Verification items for the finished model (mm, model axes). Face numbers are marked on the shaded views. A direction names the side the tool comes from. Round coordinates to 2 decimals unless told otherwise and drop trailing zeros. Order: outer loops, then holes, each group sorted by start corner. A loop starts at its lowest first (then second) coordinate and runs counter-clockwise, first axis right, second up. Notation, with made-up numbers: (88, -22) -> (130, -22) arc R8 ccw to (130, -8) -> close; hole circle Ø9 at (81, 20). An arc over 180 degrees is marked (long way). Return JSON: item names as keys, results as strings. Group by question number.
1) Tool access check on the marked faces 1 and 2. Record the directions out of +Z, -Z, +X, -X, +Y, -Y that give a thin tool (end or side, any length) a straight path to the whole face; none if there is none.
2) Scan lines: L1, parallel to X at y = -8, z = 85.5; L2, parallel to Y at x = 46.5, z = 56; L3, parallel to X at y = 4.75, z = 279.4. Record each from-to range of solid material in increasing order.
3) Section check B-B on x = 17. Enter the section's corners in (y, z).
4) Depth check by flat-ended pin: pin 1 (4 mm diameter, centred on x = 8.58, z = 279.4, fed in from -Y); pin 2 (2.5 mm diameter, centred on x = 99.38, z = 6.35, fed in from +Y); pin 3 (3.5 mm diameter, centred on x = -76, z = 267.5, fed in from +Y); pin 4 (1 mm diameter, centred on x = 61, y = -1, fed in from -Z). Enter the tip coordinate at first touch or a pass-through.
5) Section check A-A on z = 156. Enter the section's corners in (x, y), plus the area to 3 significant figures.
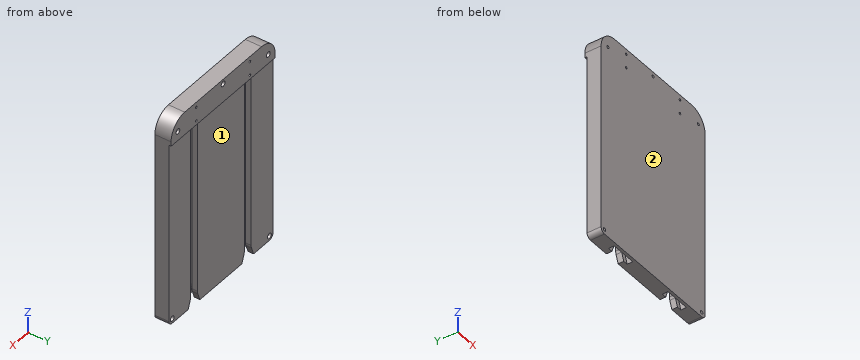
```python
from build123d import *
from OCP.BRepFilletAPI import BRepFilletAPI_MakeChamfer

# Parameters (mm, degrees)
BOSS_EXTRUDE1_DEPTH                            = 254
SKETCH2_W                                      = 194.31
SKETCH2_H                                      = 44.45
SKETCH2_W_2                                    = 35.56
SKETCH2_H_2                                    = 17.018
BOSS_EXTRUDE2_DEPTH                            = 6.35
BOSS_EXTRUDE3_DEPTH                            = 44.45
CUT_EXTRUDE1_DEPTH                             = 324.390875065
CUT_EXTRUDE1_DEPTH_BACK                        = 324.390875065
SKETCH5_R                                      = 1.524
FILLET1_R                                      = 3.175
FILLET2_R                                      = 3.175
CBORE_FOR_6_SOCKET_HEAD_CAP_SCREW1_D           = 4.3053
CBORE_FOR_6_SOCKET_HEAD_CAP_SCREW1_CBORE_D     = 7.14502
CBORE_FOR_6_SOCKET_HEAD_CAP_SCREW1_CBORE_DEPTH = 3.5052
CHAMFER1_SIZE                                  = 12.7
CHAMFER1_SIZE2                                 = 4.622421975
FILLET4_R                                      = 12.7
FILLET6_R                                      = 6.35
FILLET7_R                                      = 2.54
CUT_EXTRUDE2_DEPTH                             = 363.564005121
SKETCH13_W                                     = 19.143193239
SKETCH13_H                                     = 43.092698141
CUT_EXTRUDE3_DEPTH                             = 362.835089653
FILLET8_R                                      = 25.4
CBORE_FOR_6_SOCKET_HEAD_CAP_SCREW3_D           = 3.6576
CBORE_FOR_6_SOCKET_HEAD_CAP_SCREW3_CBORE_D     = 7.14502
CBORE_FOR_6_SOCKET_HEAD_CAP_SCREW3_CBORE_DEPTH = 3.5052
CBORE_FOR_6_SOCKET_HEAD_CAP_SCREW4_D           = 3.6576
CBORE_FOR_6_SOCKET_HEAD_CAP_SCREW4_CBORE_D     = 7.14502
CBORE_FOR_6_SOCKET_HEAD_CAP_SCREW4_CBORE_DEPTH = 3.5052


with BuildPart() as part:
    # Sketch1 → Boss-Extrude1 (new body)
    with BuildSketch(Plane.XY):
        Polygon((-88.579180599, 2.764546242), (-47.939180599, 2.764546242), (-47.939180599, -4.855453758), (-54.289180599, -4.855453758), (-54.289180599, -12.475453758), (-28.889180599, -12.475453758), (-28.889180599, -4.855453758), (-35.239180599, -4.855453758), (-35.239180599, 2.764546242), (5.400819401, 2.764546242), (5.400819401, 28.164546242), (11.750819401, 28.164546242), (11.750819401, 2.764546242), (52.390819401, 2.764546242), (52.390819401, -4.855453758), (46.040819401, -4.855453758), (46.040819401, -12.475453758), (71.440819401, -12.475453758), (71.440819401, -4.855453758), (65.090819401, -4.855453758), (65.090819401, 2.764546242), (105.730819401, 2.764546242), (105.730819401, -16.285453758), (-88.579180599, -16.285453758), align=None)
    extrude(amount=BOSS_EXTRUDE1_DEPTH)

    # Sketch2 → Boss-Extrude2 (add)
    with BuildSketch(Plane.XY.offset(254)):
        with Locations((8.575819401, 5.939546242)):
            Rectangle(SKETCH2_W, SKETCH2_H)
        with Locations((-41.589180599, 14.321546242)):
            Rectangle(SKETCH2_W_2, SKETCH2_H_2, mode=Mode.SUBTRACT)
        with Locations((58.740819401, 14.321546242)):
            Rectangle(SKETCH2_W_2, SKETCH2_H_2, mode=Mode.SUBTRACT)
    extrude(amount=BOSS_EXTRUDE2_DEPTH)

    # Sketch3 → Boss-Extrude3 (add)
    with BuildSketch(Plane.XY.offset(260.35)):
        Polygon((-88.579180599, 5.812546242), (-88.579180599, -16.285453758), (105.730819401, -16.285453758), (105.730819401, 5.812546242), (76.520819401, 5.812546242), (40.960819401, 5.812546242), (-23.809180599, 5.812546242), (-59.369180599, 5.812546242), align=None)
    extrude(amount=BOSS_EXTRUDE3_DEPTH)

    # Sketch5 → Cut-Extrude1 (cut, two sides: drawn at the far end of the back side and taken through both)
    with BuildSketch(Plane(origin=(0, 5.812546242, 0), x_dir=(1, 0, 0), z_dir=(0, 1, 0)).offset(-CUT_EXTRUDE1_DEPTH_BACK)):
        with Locations(Location((-41.589180599, -259.614, 0), (0, 0, 180))):
            Circle(SKETCH5_R)
        with Locations(Location((-41.589180599, -278.664, 0), (0, 0, 180))):
            Circle(SKETCH5_R)
        with Locations(Location((58.740819401, -259.614, 0), (0, 0, 180))):
            Circle(SKETCH5_R)
        with Locations(Location((58.740819401, -278.664, 0), (0, 0, 180))):
            Circle(SKETCH5_R)
    extrude(amount=CUT_EXTRUDE1_DEPTH + CUT_EXTRUDE1_DEPTH_BACK, mode=Mode.SUBTRACT)

    # Fillet1
    # the kernel refuses this fillet: 3.175 mm, written as the material it takes off along each edge
    with BuildSketch(Plane(origin=(5.400819401, 28.164546242, -7.9375), x_dir=(0, -1, 0), z_dir=(0, 0, 1))) as fillet1_piece_1:
        with BuildLine():
            CenterArc((FILLET1_R, FILLET1_R), FILLET1_R, 180, 90)
            Line((0, FILLET1_R), (0, 0))
            Line((0, 0), (FILLET1_R, 0))
        make_face()
    extrude(amount=261.9375, mode=Mode.SUBTRACT)
    with BuildSketch(Plane(origin=(11.750819401, 28.164546242, -7.9375), x_dir=(0, -1, 0), z_dir=(0, 0, 1))) as fillet1_piece_2:
        with BuildLine():
            CenterArc((FILLET1_R, -FILLET1_R), FILLET1_R, 90, 90)
            Line((0, -FILLET1_R), (0, 0))
            Line((0, 0), (FILLET1_R, 0))
        make_face()
    extrude(amount=261.9375, mode=Mode.SUBTRACT)

    # Fillet2
    # the kernel refuses this fillet: 3.175 mm, written as the material it adds along each edge
    # the kernel refuses this fillet: 3.175 mm, written as the material it takes off along each edge
    with BuildSketch(Plane(origin=(65.343823241, 28.164546242, 260.35), x_dir=(0, -1, 0), z_dir=(-1, 0, 0))) as fillet2_2_piece_1:
        with BuildLine():
            CenterArc((FILLET2_R, -FILLET2_R), FILLET2_R, 90, 90)
            Line((0, -FILLET2_R), (0, 0))
            Line((0, 0), (FILLET2_R, 0))
        make_face()
    extrude(amount=113.536007681, mode=Mode.SUBTRACT)
    with BuildSketch(Plane(origin=(113.668319401, 28.164546242, 260.35), x_dir=(0, -1, 0), z_dir=(-1, 0, 0)), Plane(origin=(-34.986176759, 28.164546242, 260.35), x_dir=(0, -1, 0), z_dir=(-1, 0, 0))) as fillet2_2_piece_2:
        with BuildLine():
            CenterArc((FILLET2_R, -FILLET2_R), FILLET2_R, 90, 90)
            Line((0, -FILLET2_R), (0, 0))
            Line((0, 0), (FILLET2_R, 0))
        make_face()
    extrude(amount=61.53050384, mode=Mode.SUBTRACT)
    with BuildSketch(Plane(origin=(-96.516680599, 28.164546242, 254), x_dir=(0, -1, 0), z_dir=(1, 0, 0))) as fillet2_2_piece_3_section:
        with BuildLine():
            CenterArc((FILLET2_R, -FILLET2_R), FILLET2_R, 90, 90)
            Line((0, -FILLET2_R), (0, 0))
            Line((0, 0), (FILLET2_R, 0))
        make_face()
    fillet2_2_piece_3 = extrude(amount=105.0925, mode=Mode.PRIVATE)
    fillet2_2_piece_3 = fillet2_2_piece_3 - Plane(origin=(8.575819401, 24.989546242, 254.709193206), x_dir=(0, -1, 0), z_dir=(0, 0, -1)) * Cylinder(3.175, 223, mode=Mode.PRIVATE)
    add(fillet2_2_piece_3, mode=Mode.SUBTRACT)

    # CBORE for #6 Socket Head Cap Screw1 (through all)
    with Locations(Plane(origin=(0, 2.764546242, 0), x_dir=(1, 0, 0), z_dir=(0, 1, 0))):
        with Locations((99.380819401, -6.35), (-82.229180599, -6.35)):
            CounterBoreHole(CBORE_FOR_6_SOCKET_HEAD_CAP_SCREW1_D / 2, CBORE_FOR_6_SOCKET_HEAD_CAP_SCREW1_CBORE_D / 2, CBORE_FOR_6_SOCKET_HEAD_CAP_SCREW1_CBORE_DEPTH)

    # Chamfer1: one chamfer whose edges measure the first distance from different faces: ONE call of the kernel's chamfer builder (chamfer() names one face for all edges)
    chamfer1_edges_1 = [part.edges().sort_by_distance(p)[0] for p in [
        (-47.939180599, -1.045453758, 0),
    ]]
    chamfer1_side_1 = [part.faces().sort_by_distance(p)[0] for p in [
        (-47.939180599, -1.045453758, 127),
    ]]
    chamfer1_edges_2 = [part.edges().sort_by_distance(p)[0] for p in [
        (-54.289180599, -8.665453758, 0),
    ]]
    chamfer1_side_2 = [part.faces().sort_by_distance(p)[0] for p in [
        (-54.289180599, -8.665453758, 127),
    ]]
    chamfer1_edges_3 = [part.edges().sort_by_distance(p)[0] for p in [
        (-28.889180599, -8.665453758, 0),
    ]]
    chamfer1_side_3 = [part.faces().sort_by_distance(p)[0] for p in [
        (-28.889180599, -8.665453758, 127),
    ]]
    chamfer1_edges_4 = [part.edges().sort_by_distance(p)[0] for p in [
        (-35.239180599, -1.045453758, 0),
    ]]
    chamfer1_side_4 = [part.faces().sort_by_distance(p)[0] for p in [
        (-35.239180599, -1.045453758, 127),
    ]]
    chamfer1_edges_5 = [part.edges().sort_by_distance(p)[0] for p in [
        (52.390819401, -1.045453758, 0),
    ]]
    chamfer1_side_5 = [part.faces().sort_by_distance(p)[0] for p in [
        (52.390819401, -1.045453758, 127),
    ]]
    chamfer1_edges_6 = [part.edges().sort_by_distance(p)[0] for p in [
        (46.040819401, -8.665453758, 0),
    ]]
    chamfer1_side_6 = [part.faces().sort_by_distance(p)[0] for p in [
        (46.040819401, -8.665453758, 127),
    ]]
    chamfer1_edges_7 = [part.edges().sort_by_distance(p)[0] for p in [
        (71.440819401, -8.665453758, 0),
    ]]
    chamfer1_side_7 = [part.faces().sort_by_distance(p)[0] for p in [
        (71.440819401, -8.665453758, 127),
    ]]
    chamfer1_edges_8 = [part.edges().sort_by_distance(p)[0] for p in [
        (65.090819401, -1.045453758, 0),
    ]]
    chamfer1_side_8 = [part.faces().sort_by_distance(p)[0] for p in [
        (65.090819401, -1.045453758, 127),
    ]]
    chamfer1 = BRepFilletAPI_MakeChamfer(part.part.solid().wrapped)
    for e in chamfer1_edges_1:
        chamfer1.Add(CHAMFER1_SIZE, CHAMFER1_SIZE2, e.wrapped, chamfer1_side_1[0].wrapped)  # the first distance lies on this face
    for e in chamfer1_edges_2:
        chamfer1.Add(CHAMFER1_SIZE, CHAMFER1_SIZE2, e.wrapped, chamfer1_side_2[0].wrapped)  # the first distance lies on this face
    for e in chamfer1_edges_3:
        chamfer1.Add(CHAMFER1_SIZE, CHAMFER1_SIZE2, e.wrapped, chamfer1_side_3[0].wrapped)  # the first distance lies on this face
    for e in chamfer1_edges_4:
        chamfer1.Add(CHAMFER1_SIZE, CHAMFER1_SIZE2, e.wrapped, chamfer1_side_4[0].wrapped)  # the first distance lies on this face
    for e in chamfer1_edges_5:
        chamfer1.Add(CHAMFER1_SIZE, CHAMFER1_SIZE2, e.wrapped, chamfer1_side_5[0].wrapped)  # the first distance lies on this face
    for e in chamfer1_edges_6:
        chamfer1.Add(CHAMFER1_SIZE, CHAMFER1_SIZE2, e.wrapped, chamfer1_side_6[0].wrapped)  # the first distance lies on this face
    for e in chamfer1_edges_7:
        chamfer1.Add(CHAMFER1_SIZE, CHAMFER1_SIZE2, e.wrapped, chamfer1_side_7[0].wrapped)  # the first distance lies on this face
    for e in chamfer1_edges_8:
        chamfer1.Add(CHAMFER1_SIZE, CHAMFER1_SIZE2, e.wrapped, chamfer1_side_8[0].wrapped)  # the first distance lies on this face
    add(Compound.cast(chamfer1.Shape()), mode=Mode.REPLACE)

    # Fillet4
    fillet4_edges = [part.edges().sort_by_distance(p)[0] for p in [
        (-28.889180599, -8.665453758, 12.7),
        (-35.239180599, -1.045453758, 12.7),
        (-47.939180599, -1.045453758, 12.7),
        (-54.289180599, -8.665453758, 12.7),
        (52.390819401, -1.045453758, 12.7),
        (46.040819401, -8.665453758, 12.7),
        (71.440819401, -8.665453758, 12.7),
        (65.090819401, -1.045453758, 12.7),
    ]]
    fillet(fillet4_edges, radius=FILLET4_R)

    # Fillet6
    fillet6_edges = [part.edges().sort_by_distance(p)[0] for p in [
        (105.730819401, -6.760453758, 0),
        (-88.579180599, -6.760453758, 0),
    ]]
    fillet(fillet6_edges, radius=FILLET6_R)

    # Fillet7
    fillet7_edges = [part.edges().sort_by_distance(p)[0] for p in [
        (5.400819401, 13.877046242, 0),
        (8.575819401, 28.164546242, 0),
        (11.750819401, 13.877046242, 0),
    ]]
    fillet(fillet7_edges, radius=FILLET7_R)

    # Sketch8 → Cut-Extrude2 (cut, through all)
    with BuildSketch(Plane(origin=(105.730819401, 0, 0), x_dir=(0, 0, -1), z_dir=(1, 0, 0))):
        Polygon((-254, 2.764546242), (3.999834261, 2.764546242), (3.999834261, 41.93274121), (-234.463494025, 41.93274121), (-234.463494025, 51.374436441), (-260.35, 51.374436441), (-260.35, 5.812546242), (-254, 5.812546242), align=None)
    extrude(amount=-CUT_EXTRUDE2_DEPTH, mode=Mode.SUBTRACT)

    # Sketch13 → Cut-Extrude3 (cut, through all)
    with BuildSketch(Plane(origin=(105.730819401, 0, 0), x_dir=(0, 0, -1), z_dir=(1, 0, 0))):
        with Locations((-295.228403381, 5.260895312)):
            Rectangle(SKETCH13_W, SKETCH13_H)
    extrude(amount=-CUT_EXTRUDE3_DEPTH, mode=Mode.SUBTRACT)

    # Fillet8
    fillet8_edges = [part.edges().sort_by_distance(p)[0] for p in [
        (-88.579180599, -5.236453758, 285.656806761),
        (105.730819401, -5.236453758, 285.656806761),
    ]]
    fillet(fillet8_edges, radius=FILLET8_R)

    # CBORE for #6 Socket Head Cap Screw3 (through all)
    with Locations(Plane(origin=(0, 5.812546242, 0), x_dir=(1, 0, 0), z_dir=(0, 1, 0))):
        with Locations((8.575819401, -279.4)):
            CounterBoreHole(CBORE_FOR_6_SOCKET_HEAD_CAP_SCREW3_D / 2, CBORE_FOR_6_SOCKET_HEAD_CAP_SCREW3_CBORE_D / 2, CBORE_FOR_6_SOCKET_HEAD_CAP_SCREW3_CBORE_DEPTH)

    # CBORE for #6 Socket Head Cap Screw4 (through all)
    with Locations(Plane(origin=(0, 5.812546242, 0), x_dir=(1, 0, 0), z_dir=(0, 1, 0))):
        with Locations((93.030819401, -266.606806761), (-75.879180599, -266.606806761)):
            CounterBoreHole(CBORE_FOR_6_SOCKET_HEAD_CAP_SCREW4_D / 2, CBORE_FOR_6_SOCKET_HEAD_CAP_SCREW4_CBORE_D / 2, CBORE_FOR_6_SOCKET_HEAD_CAP_SCREW4_CBORE_DEPTH)


solid = part.part
```
Check result:
{
 "1": {"face 1": "-Z, +X, -X, +Y", "face 2": "+Z, -Z, +X, -X, -Y"},
 "2": {"L1": "-88.58 to -54.29, -28.89 to 46.04, 71.44 to 105.73", "L2": "-16.29 to -12.48, -4.86 to 2.76", "L3": "-79.87 to -42.92, -40.25 to 5, 12.15 to 57.41, 60.08 to 97.03"},
 "3": {"outline": "(-16.29, 0) -> (2.76, 0) -> (2.76, 254) -> (5.81, 254) -> (5.81, 285.66) -> (-16.29, 285.66) -> close"},
 "4": {"pin 1": "y = -16.29", "pin 2": "through", "pin 3": "y = 2.31", "pin 4": "z = 254"},
 "5": {"outline": "(-88.58, -16.29) -> (105.73, -16.29) -> (105.73, 2.76) -> (65.09, 2.76) -> (65.09, -4.86) -> (71.44, -4.86) -> (71.44, -12.48) -> (46.04, -12.48) -> (46.04, -4.86) -> (52.39, -4.86) -> (52.39, 2.76) -> (-35.24, 2.76) -> (-35.24, -4.86) -> (-28.89, -4.86) -> (-28.89, -12.48) -> (-54.29, -12.48) -> (-54.29, -4.86) -> (-47.94, -4.86) -> (-47.94, 2.76) -> (-88.58, 2.76) -> close", "area": "3,120 mm^2"}
}
